```python
from build123d import *

# Parameters (mm, degrees)
EXTRUDE_1_DEPTH     = 6
CUT_EXTRUDE_1_DEPTH = 6
SKETCH_3_R          = 1.25
CUT_EXTRUDE_2_DEPTH = 8
SKETCH_4_R          = 1.25
CUT_EXTRUDE_3_DEPTH = 8
SKETCH_5_R          = 1.25
CUT_EXTRUDE_4_DEPTH = 4
FILLET_2_R          = 1


with BuildPart() as part:
    # Эскиз1 → Бобышка-Вытянуть1 (new body)
    with BuildSketch(Plane.XY):
        Polygon((0, 5), (5, 0), (22.5, 0), (33.8246732, 6.538303121), (10.464101615, 47), (7, 45), (7, 41), (0, 41), (0, 33), (3, 33), (3, 13), (0, 13), align=None)
    extrude(amount=EXTRUDE_1_DEPTH)

    # Эскиз2 → Вырез-Вытянуть1 (cut)
    with BuildSketch(Plane.XY.offset(6)):
        with BuildLine():
            Line((9.483339502, 32), (9.483339502, 13))
            Line((9.483339502, 13), (20.875644347, 13))
            ThreePointArc((20.875644347, 13), (21.741669751, 13.5), (21.741669751, 14.5))
            Line((21.741669751, 14.5), (11.349364905, 32.5))
            ThreePointArc((11.349364905, 32.5), (10.224520457, 32.965925826), (9.483339502, 32))
        make_face()
    extrude(amount=-CUT_EXTRUDE_1_DEPTH, mode=Mode.SUBTRACT)

    # Эскиз3 → Вырез-Вытянуть2 (cut)
    with BuildSketch(Plane.ZY):
        with Locations(Location((3, 37, 0), (0, 0, 270))):
            Circle(SKETCH_3_R)
        with Locations(Location((3, 9, 0), (0, 0, 270))):
            Circle(SKETCH_3_R)
    extrude(amount=-CUT_EXTRUDE_2_DEPTH, mode=Mode.SUBTRACT)

    # Эскиз4 → Вырез-Вытянуть3 (cut)
    with BuildSketch(Plane.XZ):
        with Locations(Location((13.75, 3, 0), (0, 0, 270))):
            Circle(SKETCH_4_R)
    extrude(amount=-CUT_EXTRUDE_3_DEPTH, mode=Mode.SUBTRACT)

    # Эскиз5 → Вырез-Вытянуть4 (cut)
    with BuildSketch(Plane(origin=(28.1996732, 16.281088913, 0), x_dir=(0, 0, -1), z_dir=(0.8660254037844379, 0.5000000000000014, 0))):
        with Locations(Location((-3, 32.110571585, 0), (0, 0, 90))):
            Circle(SKETCH_5_R)
        with Locations(Location((-3, -7.889428415, 0), (0, 0, 90))):
            Circle(SKETCH_5_R)
    extrude(amount=-CUT_EXTRUDE_4_DEPTH, mode=Mode.SUBTRACT)

    # Скругление2
    fillet_2_edges = [part.edges().sort_by_distance(p)[0] for p in [
        (1.5, 13, 0),
        (3, 23, 0),
        (1.5, 33, 0),
        (3.5, 41, 0),
        (7, 43, 0),
        (28.1623366, 3.26915156, 6),
        (8.732050808, 46, 0),
        (28.1623366, 3.26915156, 0),
        (2.5, 2.5, 0),
        (8.732050808, 46, 6),
        (3, 13, 3),
        (3, 33, 3),
        (7, 41, 3),
        (7, 45, 3),
        (7, 43, 6),
        (3.5, 41, 6),
        (1.5, 33, 6),
        (3, 23, 6),
        (1.5, 13, 6),
        (15.179491924, 13, 0),
        (9.483339502, 22.5, 0),
        (9.483339502, 13, 3),
        (10.224520457, 32.965925826, 0),
        (16.545517328, 23.5, 0),
        (21.741669751, 13.5, 0),
        (15.179491924, 13, 6),
        (21.741669751, 13.5, 6),
        (16.545517328, 23.5, 6),
        (10.224520457, 32.965925826, 6),
        (9.483339502, 22.5, 6),
        (2.5, 2.5, 6),
    ]]
    fillet(fillet_2_edges, radius=FILLET_2_R)


solid = part.part
```
Here's how the part is built. I have some questions about the finished solid (model axes, mm). A direction names the side the tool comes from. Coordinates: 2 decimals unless noted, no trailing zeros. One line per item, written item: value.
1) We'd pull the mould along Y, two halves only. Please class faces 1 (the flat face through (20, 23, 0)), 2 (the cylindrical face through (9.112, 45.872, 0.285)), 3 (the cylindrical face through (21.734, 13.487, 3.028)): pulls with the +Y half, pulls with the -Y half, needs draft (parallel to the pull), parting line crosses it, or undercut.
Model answer:
face 1: needs draft
face 2: pulls with the +Y half
face 3: undercut
2) I need wall thicknesses on line 1 along X through (y, z) = (6.25, 3); line 2 along Z through (x, y) = (5, 37); line 3 along Y through (x, z) = (6, 2.5). Which ranges of each line are inside material? Lowest first, please.
Model answer:
line 1: x = 0 to 12.5, 15 to 33.33
line 2: z = 0 to 1.75, 4.25 to 6
line 3: y = 0 to 7.85, 10.15 to 35.85, 38.15 to 41
3) I'm going to push flat-ended pins straight in: P1, Ø1.2, axis at y = 25.5, z = 2, coming from the +X side; P2, Ø1, axis at y = 20, z = 2, coming from the +X side; P3, Ø1, axis at y = 30, z = 4.5, coming from the -X side. Where does each tip first touch, or does it pass through?
Model answer:
P1: stops at x = 23.22
P2: stops at x = 26.34
P3: stops at x = 3
4) On a 3-axis mill with a long thin cutter (end or side, diameter ignored), from which of +Z, -Z, +X, -X, +Y, -Y can I reach the whole of each face in a straight line? I mean faces 4 (the cylindrical face through (9.2, 22.9, 5.7)), 5 (the cylindrical face through (2.958, 40.699, 0.285)), 6 (the flat face through (8.69, 42.07, 3.02)), 7 (the flat face through (9.483, 23, 3)), 8 (the flat face through (1, 33, 3)). Say none if no direction works.
Model answer:
face 4: +Z
face 5: -Z, -X, +Y
face 6: none
face 7: +Z, -Z
face 8: +Z, -Z, -X
5) Suppose I cut it at A-A on x = 3.5. State how many separate pieces and enclosed holes the cut face has, and give its area (3 significant figures).
Model answer:
separate pieces: 1
enclosed holes: 2
area: 221 mm²
